from build123d import *

# Parameters (mm, degrees)
F0_W     = 30
F0_H     = 0.843597576
F0_W_2   = 1.6
F0_H_2   = 50
F1_DEPTH = 2
F2_DEPTH = 5
F3_R     = 1


with BuildPart() as f1:
    # F0 (on Top) → F1 (new body)
    with BuildSketch(Plane.XY):
        with BuildLine():
            Line((-19, -34.5), (23, -34.5))
            ThreePointArc((23, -34.5), (23.7071067812, -34.2071067812), (24, -33.5))
            Line((24, -33.5), (24, 33.5))
            ThreePointArc((24, 33.5), (23.7071067812, 34.2071067812), (23, 34.5))
            Line((23, 34.5), (-19, 34.5))
            ThreePointArc((-19, 34.5), (-19.7071067812, 34.2071067812), (-20, 33.5))
            Line((-20, 33.5), (-20, -33.5))
            ThreePointArc((-20, -33.5), (-19.7071067812, -34.2071067812), (-19, -34.5))
        make_face()
        with Locations((2, -31.878201212)):
            Rectangle(F0_W, F0_H, mode=Mode.SUBTRACT)
        with Locations((-17, 0)):
            Rectangle(F0_W_2, F0_H_2, mode=Mode.SUBTRACT)
        with Locations((21, 0)):
            Rectangle(F0_W_2, F0_H_2, mode=Mode.SUBTRACT)
        with Locations((2, 31.878201212)):
            Rectangle(F0_W, F0_H, mode=Mode.SUBTRACT)
    extrude(amount=F1_DEPTH)

    # F0 (on Top) → F2 (join)
    with BuildSketch(Plane.XY):
        with Locations((-17, 0)):
            Rectangle(F0_W_2, F0_H_2)
        with Locations((2, 31.878201212)):
            Rectangle(F0_W, F0_H)
        with Locations((21, 0)):
            Rectangle(F0_W_2, F0_H_2)
        with Locations((2, -31.878201212)):
            Rectangle(F0_W, F0_H)
    extrude(amount=F2_DEPTH)

    # F3
    f3_edges = [f1.edges().sort_by_distance(p)[0] for p in [
        (-20, 0, 0),
        (-19.707107, -34.207107, 0),
        (2, -34.5, 0),
        (23.707107, -34.207107, 0),
        (24, 0, 0),
        (23.707107, 34.207107, 0),
        (2, 34.5, 0),
        (-19.707107, 34.207107, 0),
    ]]
    fillet(f3_edges, radius=F3_R)


solid = f1.part
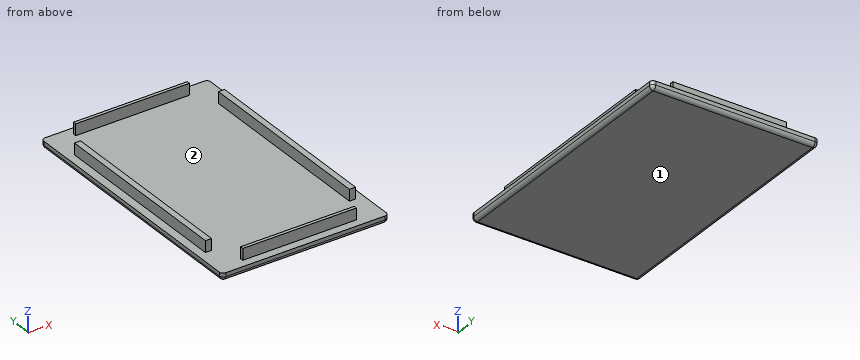
Source: CAD feature listing. Evaluate the final solid. Frame: model axes, mm. Face numbers are marked on the shaded views. Coordinates: 2 decimals unless noted, no trailing zeros. Loops run counter-clockwise (first coordinate to the right, second up) from the corner with the lowest first, then second, coordinate; pieces in that order, holes last. Notation, with made-up numbers: (81.5, 51.5) - (99.5, 51.5) arc R25 ccw to (99.5, 86.5) - close; hole circle Ø5 at (88, 35.5). An arc over 180 degrees is marked (long way). One line per question, with ' | ' between items.
1) First-contact query: P1, Ø1.3, axis at x = 20.5, z = 3, coming from the -Y side; P2, Ø1.5, axis at x = -12, y = -10.5, coming from the +Z side; P3, Ø0.9, axis at y = -5, z = 3, coming from the -X side. Flat tips, straight axial feed; report the tip coordinate or a pass-through.
Report:
P1: stops at y = -25 | P2: stops at z = 2 | P3: stops at x = -17.8
2) Section A-A, the plane z = 3.6. Return loops of the section in (x, y).
Report:
outline: (-17.8, -25) - (-16.2, -25) - (-16.2, 25) - (-17.8, 25) - close; (-13, -32.3) - (17, -32.3) - (17, -31.46) - (-13, -31.46) - close; (-13, 31.46) - (17, 31.46) - (17, 32.3) - (-13, 32.3) - close; (20.2, -25) - (21.8, -25) - (21.8, 25) - (20.2, 25) - close
3) Section B-B, the plane y = 26. Return loops of the section in (x, z), then the cut area to 3 significant figures.
Report:
outline: (-20, 1) arc R1 ccw to (-19, 0) - (23, 0) arc R1 ccw to (24, 1) - (24, 2) - (-20, 2) - close | area: 87.6 mm²
4) Line query: line 1 along Y through (x, z) = (8, 2.4); line 2 along X through (y, z) = (-20.5, 2.6); line 3 along Y through (x, z) = (-7, 0.85). Output: solid intervals per line, ascending.
Report:
line 1: y = -32.3 to -31.46, 31.46 to 32.3 | line 2: x = -17.8 to -16.2, 20.2 to 21.8 | line 3: y = -34.49 to 34.49
5) Section D-D, the plane y = 10.5. Return loops of the section in (x, z), then the cut area to 3 significant figures.
Report:
outline: (-20, 1) arc R1 ccw to (-19, 0) - (23, 0) arc R1 ccw to (24, 1) - (24, 2) - (21.8, 2) - (21.8, 5) - (20.2, 5) - (20.2, 2) - (-16.2, 2) - (-16.2, 5) - (-17.8, 5) - (-17.8, 2) - (-20, 2) - close | area: 97.2 mm²
6) Section C-C, the plane x = -12. Return loops of the section in (y, z), then the cut area to 3 significant figures.
Report:
outline: (-34.5, 1) arc R1 ccw to (-33.5, 0) - (33.5, 0) arc R1 ccw to (34.5, 1) - (34.5, 2) - (32.3, 2) - (32.3, 5) - (31.46, 5) - (31.46, 2) - (-31.46, 2) - (-31.46, 5) - (-32.3, 5) - (-32.3, 2) - (-34.5, 2) - close | area: 143 mm²
7) Pull-direction query (Y, two-part tool) for the marked faces 1 and 2; classes: released by +Y, released by -Y, zero draft, split by the parting line, or undercut.
Report:
face 1: zero draft | face 2: undercut
